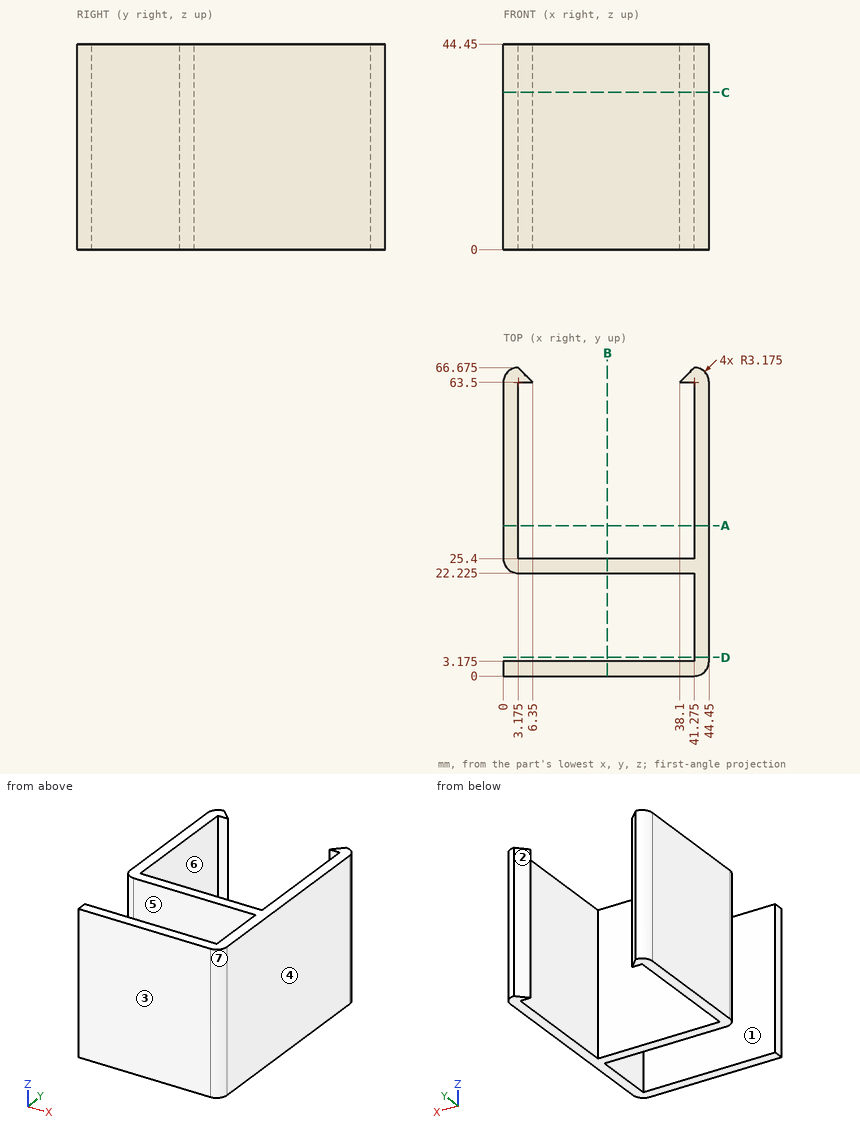
Input: dimensioned drawing with shaded views. Units: mm. Origin: part minimum x, y, z. A direction names the side the tool comes from. Round coordinates to 2 decimals unless told otherwise and drop trailing zeros. Loops run counter-clockwise (first coordinate to the right, second up) from the corner with the lowest first, then second, coordinate; pieces in that order, holes last. Notation, with made-up numbers: M 22,8.5 L 43,8.5 A11 cw 43,14.5 Z; hole C 87,5 d4. An arc over 180 degrees is marked long. One line per question, with ' | ' between items.
(1) Cut plane A-A on y = 32.5. Return the cut outline in (x, z) (3 decimals).
Check result:
outline: M 0,0 L 3.175,0 L 3.175,44.45 L 0,44.45 Z; M 41.275,0 L 44.45,0 L 44.45,44.45 L 41.275,44.45 Z
(2) Cut plane D-D on y = 4. Return the cut outline in (x, z) (3 decimals), plus the area to 3 significant figures.
Check result:
outline: M 41.275,0 L 44.45,0 L 44.45,44.45 L 41.275,44.45 Z | area: 141 mm2
(3) Pull-direction query (Y, two-part tool) for the marked faces 1, 2, 3 and 4; classes: +Y half, -Y half, draft (parallel to the pull), parting line (faces both ways), or undercut.
Check result:
face 1: undercut | face 2: +Y half | face 3: -Y half | face 4: draft
(4) Cut plane B-B on x = 22.5. Return the cut outline in (y, z) (3 decimals), plus the area to 3 significant figures.
Check result:
outline: M 0,0 L 3.175,0 L 3.175,44.45 L 0,44.45 Z; M 22.225,0 L 25.4,0 L 25.4,44.45 L 22.225,44.45 Z | area: 282 mm2
(5) Cut plane C-C on z = 34. Return the cut outline in (x, y) (3 decimals).
Check result:
outline: M 0,0 L 41.275,0 A3.175 ccw 44.45,3.175 L 44.45,63.5 A3.175 ccw 41.275,66.675 L 38.1,63.5 L 41.275,63.5 L 41.275,25.4 L 3.175,25.4 L 3.175,63.5 L 6.35,63.5 L 3.175,66.675 A3.175 ccw 0,63.5 L 0,25.4 A3.175 ccw 3.175,22.225 L 41.275,22.225 L 41.275,3.175 L 0,3.175 Z
(6) Contact query for flat-ended pins moving along their axis: P1, Ø12, axis at x = 36, z = 7, coming from the +Y side (3 decimals); P2, Ø1.5, axis at x = 39, y = 34, coming from the -Z side; P3, Ø5.5, axis at y = 14.5, z = 26.5, coming from the -X side (3 decimals); P4, Ø20.5, axis at x = 17.5, z = 17.5, coming from the +Y side. Output: stop coordinate, or through.
Check result:
P1: stops at y = 66.675 | P2: passes through | P3: stops at x = 41.275 | P4: stops at y = 25.4
(7) Material intervals for line 1 along X through (y, z) = (25.5, 23) (3 decimals); line 2 along Y through (x, z) = (37, 40.5) (3 decimals); line 3 along Y through (x, z) = (40, 40.5) (3 decimals), sorted ascending. Write a range as from..to.
Check result:
line 1: x = 0..3.175, 41.275..44.45 | line 2: y = 0..3.175, 22.225..25.4 | line 3: y = 0..3.175, 22.225..25.4, 63.5..65.4
(8) Access query for the marked faces 5, 6 and 7. Directions: +Z, -Z, +X, -X, +Y, -Y. A direction counts if a zero-diameter tool reaches every point of the face in a straight line with its end or side. Return the directions, or none.
Check result:
face 5: +Z, -Z, -X | face 6: +Z, -Z | face 7: +Z, -Z, +X, -Y
